Part model, mm, in its own coordinate system. A direction names the side the tool comes from. Round coordinates to 2 decimals unless told otherwise and drop trailing zeros. Loops run counter-clockwise (first coordinate to the right, second up) from the corner with the lowest first, then second, coordinate; pieces in that order, holes last. Notation, with made-up numbers: (11, -9.5) -> (62, -9.5) arc R13 ccw to (62, 6.5) -> close; hole circle Ø9 at (-22, 85). An arc over 180 degrees is marked (long way). Use a Markdown table: item, result. Add a question column.
Item 1: Two-plate mould, pull along Z, no slides. Class faces 1 (the face through (-1, 100, -12.7)), 2 (the face through (0, 3.175, 0)), 3 (the face through (-3, 203.2, 10)): pulls with the +Z half, pulls with the -Z half, needs draft (parallel to the pull), parting line crosses it, or undercut.
Item 2: Which spindle directions (+Z, -Z, +X, -X, +Y, -Y) get a long thin tool onto all of the face, cutting with end or side? Do faces 4 (the face through (38.1, 100, 0)), 5 (the face through (34.925, 105, 0)). Say none if no direction does.
Item 3: Cut at A-A, the plane x = -14. List the corners of the cut face in (y, z) (3 decimals).
Item 4: Cut at C-C, the plane y = 99.5. List the corners of the cut face in (x, z) (3 decimals).
Item 5: Cut at B-B, the plane z = -5. List the corners of the cut face in (x, y) (3 decimals).
Item 6: Probe line 1 (X direction, y = 15, z = 9.75); line 2 (Z direction, x = -33.5, y = 26) (3 decimals); line 3 (X direction, y = 147, z = -8.5) (3 decimals). List the from-to ranges inside material, lowest first. Write a range as [from, to].
Item 7: Flat gauge pin, fed straight in: pin 1 (12 mm diameter, centred on x = -25, y = 98.5, fed in from +Z) (3 decimals). Where does the tip first touch, or does it go through?
```python
from build123d import *

# Parameters (mm, degrees)
SKETCH1_W           = 76.2
SKETCH1_H           = 25.4
BOSS_EXTRUDE5_DEPTH = 203.2
SKETCH4_W           = 69.85
SKETCH4_H           = 19.05
CUT_EXTRUDE1_DEPTH  = 200.025
SKETCH5_W           = 63.5
SKETCH5_H           = 190.5
CUT_EXTRUDE2_DEPTH  = 8.89


with BuildPart() as part:
    # Sketch1 → Boss-Extrude5 (new body)
    with BuildSketch(Plane(origin=(0, 0, 0), x_dir=(1, 0, 0), z_dir=(0, 1, 0))):
        Rectangle(SKETCH1_W, SKETCH1_H)
    extrude(amount=BOSS_EXTRUDE5_DEPTH)

    # Sketch4 → Cut-Extrude1 (cut)
    with BuildSketch(Plane(origin=(0, 203.2, 0), x_dir=(1, 0, 0), z_dir=(0, 1, 0))):
        Rectangle(SKETCH4_W, SKETCH4_H)
    extrude(amount=-CUT_EXTRUDE1_DEPTH, mode=Mode.SUBTRACT)

    # Sketch5 → Cut-Extrude2 (cut)
    with BuildSketch(Plane.XY.offset(12.7)):
        with Locations((0, 101.6)):
            Rectangle(SKETCH5_W, SKETCH5_H)
    extrude(amount=-CUT_EXTRUDE2_DEPTH, mode=Mode.SUBTRACT)


solid = part.part
```
A:
| question | item | result |
|---|---|---|
| 1 | face 1 | pulls with the -Z half |
| 1 | face 2 | undercut |
| 1 | face 3 | needs draft |
| 2 | face 4 | +Z, -Z, +X, +Y, -Y |
| 2 | face 5 | +Y |
| 3 | outline | (0, -12.7) -> (203.2, -12.7) -> (203.2, -9.525) -> (3.175, -9.525) -> (3.175, 9.525) -> (6.35, 9.525) -> (6.35, 12.7) -> (0, 12.7) -> close; (196.85, 9.525) -> (203.2, 9.525) -> (203.2, 12.7) -> (196.85, 12.7) -> close |
| 4 | outline | (-38.1, -12.7) -> (38.1, -12.7) -> (38.1, 12.7) -> (31.75, 12.7) -> (31.75, 9.525) -> (34.925, 9.525) -> (34.925, -9.525) -> (-34.925, -9.525) -> (-34.925, 9.525) -> (-31.75, 9.525) -> (-31.75, 12.7) -> (-38.1, 12.7) -> close |
| 5 | outline | (-38.1, 0) -> (38.1, 0) -> (38.1, 203.2) -> (34.925, 203.2) -> (34.925, 3.175) -> (-34.925, 3.175) -> (-34.925, 203.2) -> (-38.1, 203.2) -> close |
| 6 | line 1 | x = [-38.1, -31.75], [31.75, 38.1] |
| 6 | line 2 | z = [-12.7, -9.525], [9.525, 12.7] |
| 6 | line 3 | x = [-38.1, -34.925], [34.925, 38.1] |
| 7 | pin 1 | stops at z = -9.525 |
